Source: CAD feature listing. Evaluate the final solid. Frame: model axes, mm. Give positions to 0.01 mm unless a question says otherwise; leave off trailing zeros. Write each loop counter-clockwise with the first axis right and the second up, starting at its lowest first coordinate (ties: lowest second). Pieces come first, ordered by that corner, then holes.
```python
from build123d import *

# Parameters (mm, degrees)
F0_R     = 1.25
F1_DEPTH = 5
F3_D     = 1.5
F3_DEPTH = 5
F3_TIP   = 0.4506454643


with BuildPart() as f1:
    # F0 (on Front) → F1 (new body, symmetric)
    with BuildSketch(Plane.XZ):
        Polygon((38.9079287648, 0.7754686598), (-26.0920712352, 0.7754686598), (-36.0920712352, -9.2245313402), (38.9079287648, -9.2245313402), (48.9079287648, 0.7754686598), align=None)
        with Locations((-6.0920712352, -4.2245313402)):
            Circle(F0_R, mode=Mode.SUBTRACT)
        with Locations((18.9079287648, -4.2245313402)):
            Circle(F0_R, mode=Mode.SUBTRACT)
    extrude(amount=F1_DEPTH, both=True)

    # F3
    with Locations(Plane(origin=(-13.4337699475, 0, 13.4337699475), x_dir=(0.7071067812, 0, 0.7071067812), z_dir=(-0.7071067812, 0, 0.7071067812))):
        with Locations((-21.4370752636, 0)):
            Hole(F3_D / 2, depth=F3_DEPTH)
            with Locations((0, 0, -(F3_DEPTH + F3_TIP / 2))):  # 118° drill point
                Cone(0, F3_D / 2, F3_TIP, mode=Mode.SUBTRACT)


solid = f1.part
```
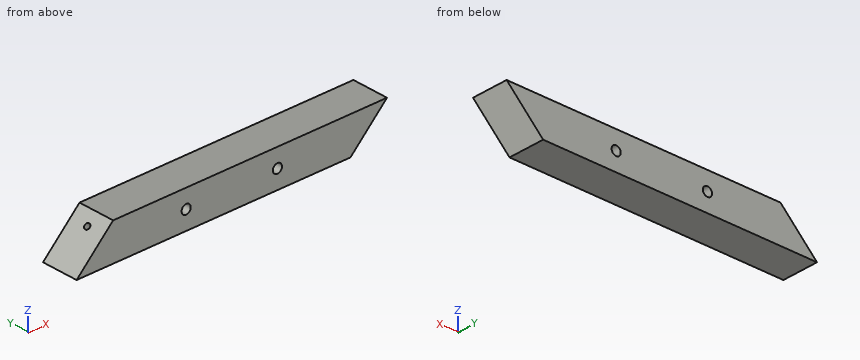
1. Section query A-A (y = 1.5). Return loops of the section in (x, z), plus the area to 3 significant figures.
2. Line query: probe 1 along X at (y, z) = (-2.5, -3.5); probe 2 along X at (y, z) = (-2.5, -3.25); probe 3 along X at (y, z) = (0.25, -1.5). Output: solid intervals per line, ascending.
3. Pin query (flat end, axial travel): P1, Ø2, axis at y = -1, z = -4, coming from the +X side. Return the tip coordinate at first contact, or that it passes through.
4. Section query B-B (z = -8). Return loops of the section in (x, y).
The answers:
1. outline: (-36.09, -9.22) - (38.91, -9.22) - (48.91, 0.78) - (-26.09, 0.78) - close; hole circle Ø2.5 at (-6.09, -4.22); hole circle Ø2.5 at (18.91, -4.22)
1. area: 740 mm2
2. probe 1: x = -30.37 to -7.11, -5.07 to 17.89, 19.93 to 44.63
2. probe 2: x = -30.12 to -6.87, -5.31 to 18.13, 19.69 to 44.88
2. probe 3: x = -27.82 to 46.63
3. P1: stops at x = 45.13
4. outline: (-34.87, -5) - (40.13, -5) - (40.13, 5) - (-34.87, 5) - close
